Build history of the part. All positions in model axes, mm. Face numbers are marked on the shaded views. A direction names the side the tool comes from. Round coordinates to 2 decimals unless told otherwise and drop trailing zeros. Write each loop counter-clockwise with the first axis right and the second up, starting at its lowest first coordinate (ties: lowest second). Pieces come first, ordered by that corner, then holes. Notation, with made-up numbers: (9, 53.5) - (31, 53.5) arc R18 cw to (31, 58.5) - close; hole circle Ø11 at (-17, 41.25). An arc over 180 degrees is marked (long way). Answer as a JSON object with one key per item and string values. Group by question number.
Item 1: Slice it at A-A, the plane y = 0. List the corners of the cut face in (x, z).
Item 2: Which spindle directions (+Z, -Z, +X, -X, +Y, -Y) get a long thin tool onto all of the face, cutting with end or side? Do the marked faces 1 and 2. Say none if no direction does.
Item 3: Probe line 1 (Z direction, x = 2.75, y = 0); line 2 (Z direction, x = 7, y = 0); line 3 (X direction, y = -0.5, z = -4.25). List the from-to ranges inside material, lowest first. Write a range as from..to.
Item 4: Flat gauge pins, fed straight in: pin 1 (3 mm diameter, centred on x = 2, y = -3, fed in from +Z); pin 2 (2 mm diameter, centred on x = 9.5, z = 3.5, fed in from -Y); pin 3 (3 mm diameter, centred on x = 5, y = -4, fed in from +Z). Where does each tip first touch, or does it go through?
Item 5: Slice it at C-C, the plane x = 2. List the corners of the cut face in (y, z), then the cut area to 3 significant figures.
Item 6: Slice it at D-D, the plane z = 4. List the corners of the cut face in (x, y).
Autodesk Inventor part; units mm, degrees
ref_plane "YZ Plane" through (0, 0, 0) normal (1, 0, 0) x (0, 1, 0)
ref_plane "XZ Plane" through (0, 0, 0) normal (0, 1, 0) x (-1, 0, 0)
ref_plane "XY Plane" through (0, 0, 0) normal (0, 0, 1) x (1, 0, 0)
sketch "Sketch1" plane through (0, 0, 0) normal (0, 0, 1) x (1, 0, 0)
  line L0 (0, 0) -> (4, 0)
  line L1 (4, 0) -> (4, 3)
  line L2 (4, 3) -> (0, 3)
  line L3 (0, 3) -> (0, 0)
  line L4 (4, 0) -> (12, 0)
  line L5 (12, 0) -> (12, 5)
  line L6 (12, 5) -> (4, 5)
  line L7 (4, 5) -> (4, 0)
  line L8 (0, 0) -> (12, 0)
  dimension "d0" = 5
  dimension "d1" = 3
  dimension "d2" = 4
  dimension "d3" = 8
revolve "Revolution1" add sketch "Sketch1" angle 360 about axis through (4, 0, 0) along (1, 0, 0)
fillet "Fillet1" radius 0.5 1 edges at (4, -3, 0)
chamfer "Chamfer1" distance 0.5 angle 45 1 edges at (0, -3, 0)
sketch "Sketch2" plane through (0, 0, 0) normal (-1, 0, 0) x (0, 0, 1)
  circle A0 centre (0, 0) radius 3
  point P0 (0, 0)
  point P1 (0, 0)
hole "Hole1" at (0, 0, 0) direction (1, 0, 0) diameter 2.459 end through all
properties part number "Selection_Lever Mount Piece" material "Aluminum 6061"
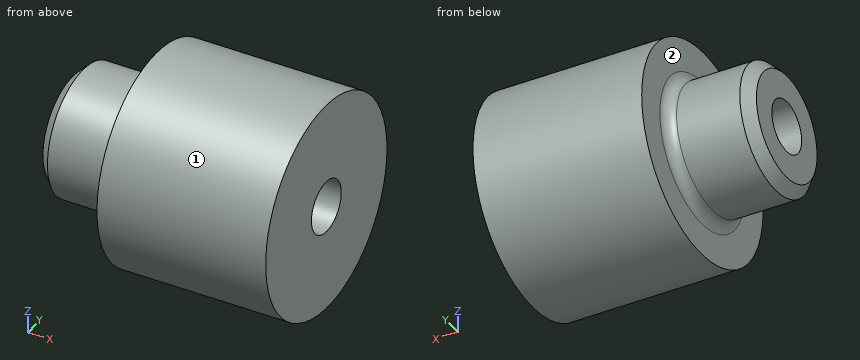
Geometry says:
{
 "1": {"outline": "(0, -2.5) - (0.5, -3) - (3.5, -3) arc R0.5 cw to (4, -3.5) - (4, -5) - (12, -5) - (12, -1.23) - (0, -1.23) - close; (0, 1.23) - (12, 1.23) - (12, 5) - (4, 5) - (4, 3.5) arc R0.5 cw to (3.5, 3) - (0.5, 3) - (0, 2.5) - close"},
 "2": {"face 1": "+X, -X", "face 2": "-X"},
 "3": {"line 1": "z = -3..-1.23, 1.23..3", "line 2": "z = -5..-1.23, 1.23..5", "line 3": "x = 4..12"},
 "4": {"pin 1": "stops at z = 2.6", "pin 2": "stops at y = -4.33", "pin 3": "stops at z = 4.33"},
 "5": {"outline": "circle Ø6 at (0, 0); hole circle Ø2.46 at (0, 0)", "area": "23.5 mm^2"},
 "6": {"outline": "(4, -3) - (12, -3) - (12, 3) - (4, 3) - close"}
}
